Here's how the part is built. I have some questions about the finished solid (model axes, mm). Face numbers are marked on the shaded views. Round coordinates to 2 decimals unless told otherwise and drop trailing zeros. Write each loop counter-clockwise with the first axis right and the second up, starting at its lowest first coordinate (ties: lowest second). Pieces come first, ordered by that corner, then holes. Notation, with made-up numbers: M -24,36 L 8,36 A15 ccw 8,41 Z; hole C 68.5,53 d7. An arc over 180 degrees is marked long. Use a Markdown table: item, result. Add a question column.
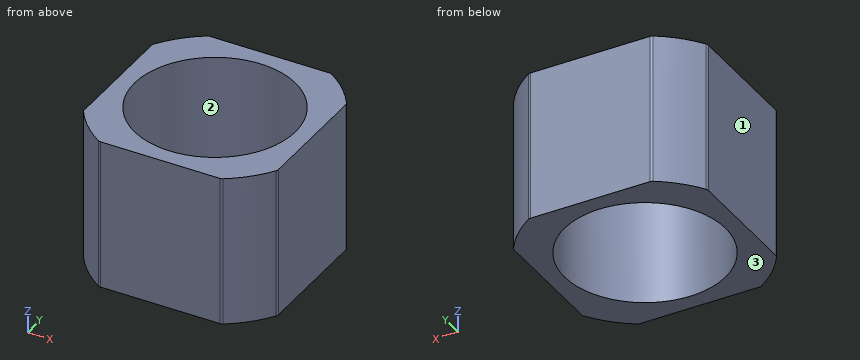
```python
from build123d import *

# Parameters (mm, degrees)
CROQUIS1_W              = 42.3
CROQUIS1_H              = 42.3
SALIENTE_EXTRUIR1_DEPTH = 32.8
SKETCH1_R               = 29.910616844
SKETCH1_R_2             = 25
CUT_EXTRUDE1_DEPTH      = 33.8
FILLET1_R               = 1
SKETCH2_R               = 17.5
CUT_EXTRUDE2_DEPTH      = 33.8


with BuildPart() as part:
    # Croquis1 → Saliente-Extruir1 (new body)
    with BuildSketch(Plane.XY):
        Rectangle(CROQUIS1_W, CROQUIS1_H)
    extrude(amount=SALIENTE_EXTRUIR1_DEPTH)

    # Sketch1 → Cut-Extrude1 (cut, through all)
    with BuildSketch(Plane.XY.offset(32.8)):
        Circle(SKETCH1_R)
        Circle(SKETCH1_R_2, mode=Mode.SUBTRACT)
    extrude(amount=-CUT_EXTRUDE1_DEPTH, mode=Mode.SUBTRACT)

    # Fillet1
    fillet1_edges = [part.edges().sort_by_distance(p)[0] for p in [
        (21.15, -13.329572386, 16.4),
        (21.15, 13.329572386, 16.4),
        (13.329572386, 21.15, 16.4),
        (-13.329572386, 21.15, 16.4),
        (-21.15, 13.329572386, 16.4),
        (-21.15, -13.329572386, 16.4),
        (-13.329572386, -21.15, 16.4),
        (13.329572386, -21.15, 16.4),
    ]]
    fillet(fillet1_edges, radius=FILLET1_R)

    # Sketch2 → Cut-Extrude2 (cut, through all)
    with BuildSketch(Plane.XY.offset(32.8)):
        Circle(SKETCH2_R)
    extrude(amount=-CUT_EXTRUDE2_DEPTH, mode=Mode.SUBTRACT)


solid = part.part
```
Item 1: Imagine slicing it at A-A on y = 0. List the corners of the cut face in (x, z) for me, plus the area to 3 significant figures.
Item 2: If we mould it in two halves opening along X, with no side actions, what happens to the marked faces 1, 2 and 3? For each: +X half, -X half, draft (parallel to the pull), parting line (faces both ways), or undercut.
Item 3: Imagine slicing it at B-B on z = 14.5. List the corners of the cut face in (x, y) for me, plus the area to 3 significant figures.
Item 4: I need wall thicknesses on probe 1 along Y at (x, z) = (0, 12); probe 2 along X at (y, z) = (-13.5, 27); probe 3 along X at (y, z) = (3, 30.5). Which ranges of each line are inside material? Lowest first, please. Write a range as from..to.
Item 5: For pin 1 Ø5 at (x, y) = (-7, 11) entering from +Z; pin 2 Ø1.5 at (x, z) = (14.5, 19.5) entering from +Y; pin 3 Ø6 at (x, z) = (-14.5, 22.5) entering from -Y, each with a flat end and sliding along its axis, tell me the tip position at first contact or that it passes through.
The answers:
| question | item | result |
|---|---|---|
| 1 | outline | M -21.15,0 L -17.5,0 L -17.5,32.8 L -21.15,32.8 Z; M 17.5,0 L 21.15,0 L 21.15,32.8 L 17.5,32.8 Z |
| 1 | area | 239 mm² |
| 2 | face 1 | -X half |
| 2 | face 2 | undercut |
| 2 | face 3 | draft |
| 3 | outline | M -21.15,-13.04 A1 ccw -20.99,-13.58 A25 ccw -13.58,-20.99 A1 ccw -13.04,-21.15 L 13.04,-21.15 A1 ccw 13.58,-20.99 A25 ccw 20.99,-13.58 A1 ccw 21.15,-13.04 L 21.15,13.04 A1 ccw 20.99,13.58 A25 ccw 13.58,20.99 A1 ccw 13.04,21.15 L -13.04,21.15 A1 ccw -13.58,20.99 A25 ccw -20.99,13.58 A1 ccw -21.15,13.04 Z; hole C 0,0 d35 |
| 3 | area | 723 mm² |
| 4 | probe 1 | -21.15..-17.5, 17.5..21.15 |
| 4 | probe 2 | -21.04..-11.14, 11.14..21.04 |
| 4 | probe 3 | -21.15..-17.24, 17.24..21.15 |
| 5 | pin 1 | through |
| 5 | pin 2 | y = 20.88 |
| 5 | pin 3 | y = -21.15 |
